Can you work these out from the model? Positions are in its coordinate system, mm. Face numbers are marked on the shaded views. A direction names the side the tool comes from. Give positions to 0.01 mm unless a question says otherwise; leave off trailing zeros. Loops run counter-clockwise (first coordinate to the right, second up) from the corner with the lowest first, then second, coordinate; pieces in that order, holes last. Notation, with made-up numbers: M 62.25,66.5 L 82.25,66.5 A28 cw 82.25,92.5 Z; hole C 80.25,24.25 d7. An arc over 180 degrees is marked long. Answer as a JSON object with one key per item and string values.
```python
from build123d import *
from build123d.topology import SkipClean

# Parameters (mm, degrees)
EXTRUDE_1_DEPTH     = 5
SKETCH_2_R          = 10
EXTRUDE_2_DEPTH     = 15
SKETCH_3_R          = 4
EXTRUDE_3_DEPTH     = 6
SKETCH_4_R          = 5
SKETCH_4_R_2        = 4
EXTRUDE_4_DEPTH     = 1
CHAMFER_1_SIZE      = 0.5
SKETCH_6_R          = 1.3
CUT_EXTRUDE_2_DEPTH = 6
SKETCH_11_R         = 2.2
CUT_EXTRUDE_7_DEPTH = 10
CUT_EXTRUDE_START   = -5
CUT_EXTRUDE_8_DEPTH = 5
SKETCH_14_R         = 5
CUT_EXTRUDE_9_DEPTH = 3
EXTRUDE_START       = -1
SKETCH_15_R         = 10
EXTRUDE_5_DEPTH     = 1
FILLET_1_R          = 2
SKETCH_16_W         = 4.663078912
SKETCH_16_H         = 1.2
EXTRUDE_6_DEPTH     = 4
EXTRUDE_START_2     = 1
EXTRUDE_7_DEPTH     = 1
EXTRUDE_8_DEPTH     = 3


with BuildPart() as part:
    # 草图1 → 凸台-拉伸1 (new body)
    with BuildSketch(Plane.XY):
        with BuildLine():
            Line((52.673076923, 6.967565389), (1.153846154, 11.94439781))
            ThreePointArc((1.153846154, 11.94439781), (-12, 0), (1.153846154, -11.94439781))
            Line((1.153846154, -11.94439781), (52.673076923, -6.967565389))
            ThreePointArc((52.673076923, -6.967565389), (59, 0), (52.673076923, 6.967565389))
        make_face()
    extrude(amount=EXTRUDE_1_DEPTH)

    # 草图2 → 凸台-拉伸2 (add)
    with BuildSketch(Plane.XY.offset(5)):
        Circle(SKETCH_2_R)
    extrude(amount=EXTRUDE_2_DEPTH)

    # 草图3 → 凸台-拉伸3 (add)
    with BuildSketch(Plane(origin=(0, 0, 0), x_dir=(-1, 0, 0), z_dir=(0, 0, -1))):
        with Locations((-52, 0)):
            Circle(SKETCH_3_R)
    extrude(amount=EXTRUDE_3_DEPTH)

    # 草图4 → 凸台-拉伸4 (add)
    with BuildSketch(Plane(origin=(0, 0, 0), x_dir=(-1, 0, 0), z_dir=(0, 0, -1))):
        with Locations(Location((-52, 0, 0), (0, 0, 180))):
            Circle(SKETCH_4_R)
        with Locations((-52, 0)):
            Circle(SKETCH_4_R_2, mode=Mode.SUBTRACT)
    extrude(amount=EXTRUDE_4_DEPTH)

    # 倒角1
    chamfer_1_edges = [part.edges().sort_by_distance(p)[0] for p in [
        (-10, 0, 20),
        (56, 0, -6),
        (47, 0, -1),
    ]]
    chamfer(chamfer_1_edges, length=CHAMFER_1_SIZE)

    # 草图6 → 切除-拉伸2 (cut)
    with BuildSketch(Plane.XY.offset(20)):
        with Locations((0, 7)):
            Circle(SKETCH_6_R)
        with Locations((7, 0)):
            Circle(SKETCH_6_R)
        with Locations((0, -7)):
            Circle(SKETCH_6_R)
        with Locations((-7, 0)):
            Circle(SKETCH_6_R)
    extrude(amount=-CUT_EXTRUDE_2_DEPTH, mode=Mode.SUBTRACT)

    # 草图11 → 切除-拉伸7 (cut)
    with BuildSketch(Plane(origin=(0, 0, -6), x_dir=(-1, 0, 0), z_dir=(0, 0, -1))):
        with Locations((-52, 0)):
            Circle(SKETCH_11_R)
    extrude(amount=-CUT_EXTRUDE_7_DEPTH, mode=Mode.SUBTRACT)

    # 草图12 → 切除-拉伸8 (cut)
    with BuildSketch(Plane.XY.offset(5).offset(CUT_EXTRUDE_START)):
        with BuildLine():
            Line((47.604489244, 5.447888141), (7.564052776, 9.315852382))
            ThreePointArc((7.564052776, 9.315852382), (10.834404305, 5.159038995), (12, 0))
            ThreePointArc((12, 0), (10.834404305, -5.159038995), (7.564052776, -9.315852382))
            Line((7.564052776, -9.315852382), (47.604489244, -5.447888141))
            ThreePointArc((47.604489244, -5.447888141), (45, 0), (47.604489244, 5.447888141))
        make_face()
    extrude(amount=CUT_EXTRUDE_8_DEPTH, mode=Mode.SUBTRACT)

    # 草图14 → 切除-拉伸9 (cut)
    # profile 1 of 2: a face of its own
    with BuildSketch(Plane(origin=(0, 0, 0), x_dir=(-1, 0, 0), z_dir=(0, 0, -1))):
        with BuildLine():
            Line((-52.673076923, 6.967565389), (-44.130557544, 7.792785152))
            ThreePointArc((-44.130557544, 7.792785152), (-63.075, 0), (-44.130557544, -7.792785152))
            Line((-44.130557544, -7.792785152), (-52.673076923, -6.967565389))
            ThreePointArc((-52.673076923, -6.967565389), (-59, 0), (-52.673076923, 6.967565389))
        make_face()
    # profile 2 of 2: a face of its own
    with BuildSketch(Plane(origin=(0, 0, 0), x_dir=(-1, 0, 0), z_dir=(0, 0, -1))):
        with BuildLine():
            ThreePointArc((-44.130557544, -7.792785152), (-41.757693126, -4.213166849), (-40.925, 0))
            ThreePointArc((-40.925, 0), (-41.757693126, 4.213166849), (-44.130557544, 7.792785152))
            Line((-44.130557544, 7.792785152), (-52.673076923, 6.967565389))
            ThreePointArc((-52.673076923, 6.967565389), (-59, 0), (-52.673076923, -6.967565389))
            Line((-52.673076923, -6.967565389), (-44.130557544, -7.792785152))
        make_face()
        with Locations((-52, 0)):
            Circle(SKETCH_14_R, mode=Mode.SUBTRACT)
    extrude(amount=-CUT_EXTRUDE_9_DEPTH, mode=Mode.SUBTRACT)

    # 草图15 → 凸台-拉伸5 (add)
    # profile 1 of 2: a face of its own
    with SkipClean():  # the faces are left unmerged after this step: merging them gives an invalid solid
        with BuildSketch(Plane.XY.offset(5).offset(EXTRUDE_START)):
            with BuildLine():
                ThreePointArc((1.153846154, 11.94439781), (-12, 0), (1.153846154, -11.94439781))
                Line((1.153846154, -11.94439781), (52.673076923, -6.967565389))
                ThreePointArc((52.673076923, -6.967565389), (59, 0), (52.673076923, 6.967565389))
                Line((52.673076923, 6.967565389), (1.153846154, 11.94439781))
            make_face()
            Circle(SKETCH_15_R, mode=Mode.SUBTRACT)
            with BuildLine():
                ThreePointArc((7.564052776, -9.315852382), (12, 0), (7.564052776, 9.315852382))
                Line((7.564052776, 9.315852382), (47.604489244, 5.447888141))
                ThreePointArc((47.604489244, 5.447888141), (45, 0), (47.604489244, -5.447888141))
                Line((47.604489244, -5.447888141), (7.564052776, -9.315852382))
            make_face(mode=Mode.SUBTRACT)
        # profile 2 of 2: a face of its own
        with BuildSketch(Plane.XY.offset(5).offset(EXTRUDE_START)):
            with BuildLine():
                Line((47.604489244, 5.447888141), (7.564052776, 9.315852382))
                ThreePointArc((7.564052776, 9.315852382), (12, 0), (7.564052776, -9.315852382))
                Line((7.564052776, -9.315852382), (47.604489244, -5.447888141))
                ThreePointArc((47.604489244, -5.447888141), (45, 0), (47.604489244, 5.447888141))
            make_face()
        extrude(amount=EXTRUDE_5_DEPTH)
    add(part.part.scale(1), mode=Mode.REPLACE)  # the faces are merged on a copy

    # 圆角1
    # the kernel refuses this fillet: 2 mm, written as the material it takes off along each edge
    with BuildSketch(Plane(origin=(44.130557544, -7.792785152, -8.249501326), x_dir=(-0.9953664842005795, -0.09615384615384645, 0), z_dir=(0, 0, 1)), Plane(origin=(44.130557544, 7.792785152, 3), x_dir=(-0.9953664842005796, 0.09615384615384538, 0), z_dir=(0, 0, -1))) as fillet_1_piece_1:
        with BuildLine():
            CenterArc((3.29980053, -2), FILLET_1_R, 90, 90)
            ThreePointArc((1.29980053, -2), (0.703900692, -0.964905108), (0, 0))
            Line((0, 0), (3.29980053, 0))
        make_face()
    extrude(amount=11.249501326, mode=Mode.SUBTRACT)

    # 草图16 → 切除-旋转1 (revolve, cut)
    with BuildSketch(Plane(origin=(0, 0, 0), x_dir=(1, 0, 0), z_dir=(0, 1, 0))):
        with Locations((11.581539456, -17.6)):
            Rectangle(SKETCH_16_W, SKETCH_16_H)
    revolve(axis=Axis((0, 0, 20), (0, 0, -1)), mode=Mode.SUBTRACT)

    # 草图17 → 凸台-拉伸6 (add)
    with BuildSketch(Plane(origin=(0, 0, 4), x_dir=(-1, 0, 0), z_dir=(0, 0, -1))):
        with BuildLine():
            Line((-7.564052776, 9.315852382), (-42.644471967, 5.927033004))
            ThreePointArc((-42.644471967, 5.927033004), (-40.925, 0), (-42.644471967, -5.927033004))
            Line((-42.644471967, -5.927033004), (-7.564052776, -9.315852382))
            ThreePointArc((-7.564052776, -9.315852382), (-12, 0), (-7.564052776, 9.315852382))
        make_face()
        with BuildLine():
            Line((-38.644471967, 2.294818465), (-38.644471967, -2.294818465))
            Line((-38.644471967, -2.294818465), (-15.340593905, -4.546006888))
            ThreePointArc((-15.340593905, -4.546006888), (-16, 0), (-15.340593905, 4.546006888))
            Line((-15.340593905, 4.546006888), (-38.644471967, 2.294818465))
        make_face(mode=Mode.SUBTRACT)
    extrude(amount=EXTRUDE_6_DEPTH)

    # 草图18 → 凸台-拉伸7 (add)
    with BuildSketch(Plane(origin=(0, 0, 4), x_dir=(-1, 0, 0), z_dir=(0, 0, -1)).offset(EXTRUDE_START_2)):
        with BuildLine():
            Line((-42.644471967, 5.927033004), (-47.604489244, 5.447888141))
            ThreePointArc((-47.604489244, 5.447888141), (-45, 0), (-47.604489244, -5.447888141))
            Line((-47.604489244, -5.447888141), (-42.644471967, -5.927033004))
            ThreePointArc((-42.644471967, -5.927033004), (-40.925, 0), (-42.644471967, 5.927033004))
        make_face()
    extrude(amount=-EXTRUDE_7_DEPTH)

    # 草图19 → 凸台-拉伸8 (add)
    with BuildSketch(Plane.XY.offset(5)):
        with BuildLine():
            Line((28.521899702, -9.30060414), (52.673076923, -6.967565389))
            ThreePointArc((52.673076923, -6.967565389), (59, 0), (52.673076923, 6.967565389))
            Line((52.673076923, 6.967565389), (28.521899702, 9.30060414))
            ThreePointArc((28.521899702, 9.30060414), (30, 0), (28.521899702, -9.30060414))
        make_face()
    extrude(amount=EXTRUDE_8_DEPTH)


solid = part.part
```
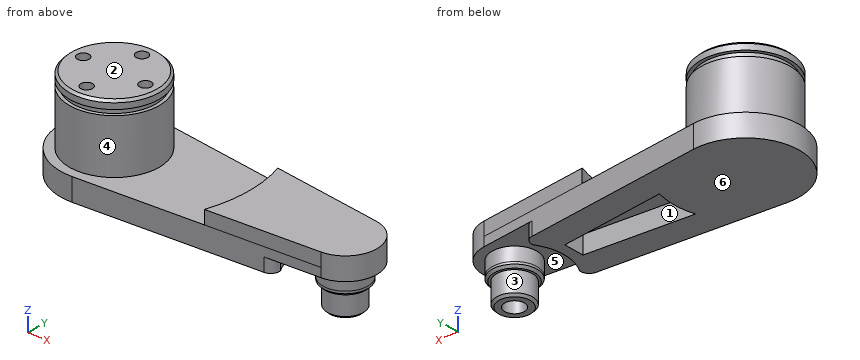
1) Suppose I cut it at B-B, the plane x = 52. Write out the boundary of the cut face in (y, z).
Answer list:
{"outline": "M -7.03,3 L -5,3 L -5,-0.5 L -4.5,-1 L -4,-1 L -4,-5.5 L -3.5,-6 L -2.2,-6 L -2.2,4 L 2.2,4 L 2.2,-6 L 3.5,-6 L 4,-5.5 L 4,-1 L 4.5,-1 L 5,-0.5 L 5,3 L 7.03,3 L 7.03,8 L -7.03,8 Z"}
2) Please list where these lines run through material, in increasing order: line 1 along Y through (x, z) = (0, 16.55); line 2 along Z through (x, y) = (9.5, -0.25); line 3 along Z through (x, y) = (6.5, -6.5). Write a range as from..to.
Answer list:
{"line 1": "-10..-8.3, -5.7..5.7, 8.3..10", "line 2": "0..17, 18.2..20", "line 3": "0..20"}
3) Suppose I cut it at A-A, the plane x = 0. Write out the boundary of the cut face in (y, z).
Answer list:
{"outline": "M -12,0 L 12,0 L 12,5 L 10,5 L 10,17 L 9.25,17 L 9.25,18.2 L 10,18.2 L 10,19.5 L 9.5,20 L 8.3,20 L 8.3,14 L 5.7,14 L 5.7,20 L -5.7,20 L -5.7,14 L -8.3,14 L -8.3,20 L -9.5,20 L -10,19.5 L -10,18.2 L -9.25,18.2 L -9.25,17 L -10,17 L -10,5 L -12,5 Z"}
4) For the marked faces 4, 5 and 6, which set-ups out of +Z, -Z, +X, -X, +Y, -Y let a thin tool reach every point of the face, with its end or its side?
Answer list:
{"face 4": "+Z", "face 5": "-Z", "face 6": "-Z, -X, +Y, -Y"}
5) Will these pins go through, and if not, where does the flat tip stop? pin 1 Ø2 at (x, y) = (52, -0.5) entering from -Z; pin 2 Ø3 at (x, y) = (-7, 0) entering from -Z; pin 3 Ø1 at (y, z) = (3.5, 17) entering from +X; pin 4 Ø12 at (x, z) = (51.5, 15.5) entering from -Y.
Answer list:
{"pin 1": "z = 4", "pin 2": "z = 0", "pin 3": "x = 9.54", "pin 4": "through"}
6) If we mould it in two halves opening along X, with no side actions, what happens to the marked faces 1, 2 and 3? For each: +X half, -X half, draft (parallel to the pull), parting line (faces both ways), or undercut.
Answer list:
{"face 1": "undercut", "face 2": "draft", "face 3": "parting line"}
